Here's how the part is built. I have some questions about the finished solid (model axes, mm). Face numbers are marked on the shaded views. A direction names the side the tool comes from. Give positions to 0.01 mm unless a question says otherwise; leave off trailing zeros. Loops run counter-clockwise (first coordinate to the right, second up) from the corner with the lowest first, then second, coordinate; pieces in that order, holes last. Notation, with made-up numbers: M 4.25,36 L 8.25,36 A20 cw 8.25,67 Z; hole C 3.25,-32 d11. An arc over 180 degrees is marked long. Answer as CSV lines item,"result". Start each with the question number.
Item 1: I want a section at B-B on y = 6.5. List the corners of the cut face in (x, z) for me, plus the area to 3 significant figures.
Item 2: For the marked faces 4, 5 and 6, which set-ups out of +Z, -Z, +X, -X, +Y, -Y let a thin tool reach every point of the face, with its end or its side?
Item 3: I want a section at A-A on z = 2.5. List the corners of the cut face in (x, y) for me, plus the area to 3 significant figures.
Item 4: If I drill on line 1 along Y through (x, z) = (-17, 13.25); line 2 along Y through (x, z) = (2, 10.25); line 3 along X through (y, z) = (-3, 6.5), over which ranges is the centre line in solid material (lowest first)? Write a range as from..to.
Item 5: I want a section at C-C on x = -17. List the corners of the cut face in (y, z) for me.
Item 6: I want a section at D-D on y = -7. List the corners of the cut face in (x, z) for me, plus the area to 3 significant figures.
Item 7: If we mould it in two halves opening along Z, with no side actions, what happens to the marked faces 1, 2 and 3? For each: released by +Z, released by -Z, zero draft, split by the parting line, or undercut.
Item 8: Will these pins go through, and if not, where does the flat tip stop? P1, Ø5, axis at x = 27.5, z = 13, coming from the -Y side; P2, Ø6.5, axis at y = 3.5, z = 8, coming from the +X side; P3, Ø12, axis at x = 29.5, y = -25, coming from the -Z side.
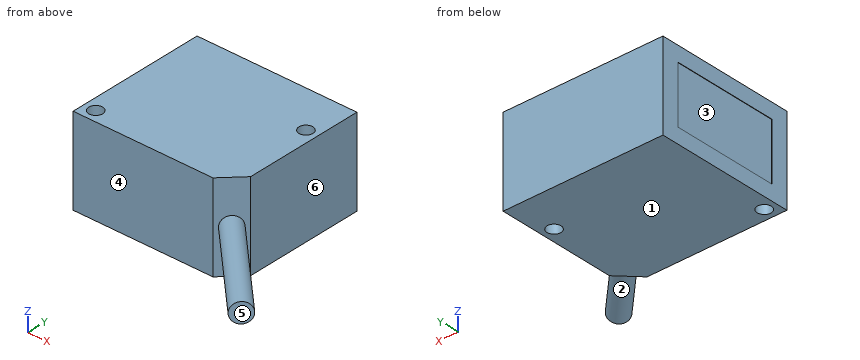
from build123d import *

# Parameters (mm, degrees)
SKETCH_1_W          = 40
SKETCH_1_H          = 35
EXTRUDE_1_DEPTH     = 22
SKETCH_2_R          = 1.75
CUT_EXTRUDE_1_DEPTH = 35.5
CHAMFER_1_SIZE      = 5
SKETCH_3_R          = 2.5
EXTRUDE_2_DEPTH     = 30
SKETCH_4_W          = 14.42354322
SKETCH_4_H          = 26.54144869
CUT_EXTRUDE_2_DEPTH = 0.1


with BuildPart() as part:
    # 草图1 → 凸台-拉伸1 (new body)
    with BuildSketch(Plane.XY):
        Rectangle(SKETCH_1_W, SKETCH_1_H)
    extrude(amount=EXTRUDE_1_DEPTH)

    # 草图2 → 切除-拉伸1 (cut, through all)
    with BuildSketch(Plane.XY.offset(22)):
        with Locations((17, 6.5)):
            Circle(SKETCH_2_R)
        with Locations((-17, -14.5)):
            Circle(SKETCH_2_R)
    extrude(amount=-CUT_EXTRUDE_1_DEPTH, mode=Mode.SUBTRACT)

    # 倒角1
    chamfer_1_edges = [part.edges().sort_by_distance(p)[0] for p in [
        (20, -17.5, 11),
    ]]
    chamfer(chamfer_1_edges, length=CHAMFER_1_SIZE)

    # 草图3 → 凸台-拉伸2 (add)
    with BuildSketch(Plane(origin=(16.25, -16.25, 0), x_dir=(0, 0, -1), z_dir=(0.7071067811865467, -0.7071067811865485, 0))):
        with Locations(Location((-11, 1.767766953, 0), (0, 0, 90))):
            Circle(SKETCH_3_R)
    extrude(amount=EXTRUDE_2_DEPTH)

    # 草图4 → 切除-拉伸2 (cut)
    with BuildSketch(Plane.ZY.offset(20)):
        with Locations((11, 0)):
            Rectangle(SKETCH_4_W, SKETCH_4_H)
    extrude(amount=-CUT_EXTRUDE_2_DEPTH, mode=Mode.SUBTRACT)


solid = part.part
Result:
1,outline,"M -20,0 L 15.25,0 L 15.25,22 L -20,22 L -20,18.21 L -19.9,18.21 L -19.9,3.79 L -20,3.79 Z; M 18.75,0 L 20,0 L 20,22 L 18.75,22 Z"
1,area,"802 mm^2"
2,face 4,"+Z, -Z, -X, -Y"
2,face 5,"+Z, -Z, +X, -Y"
2,face 6,"+Z, -Z, +X, +Y"
3,outline,"M -20,-17.5 L 15,-17.5 L 20,-12.5 L 20,17.5 L -20,17.5 Z; hole C -17,-14.5 d3.5; hole C 17,6.5 d3.5"
3,area,"1,370 mm^2"
4,line 1,"-17.5..-16.25, -12.75..17.5"
4,line 2,"-17.5..17.5"
4,line 3,"-19.9..20"
5,outline,"M -17.5,0 L -16.25,0 L -16.25,22 L -17.5,22 Z; M -12.75,0 L 17.5,0 L 17.5,22 L -12.75,22 Z"
6,outline,"M -20,0 L 20,0 L 20,22 L -20,22 L -20,18.21 L -19.9,18.21 L -19.9,3.79 L -20,3.79 Z"
6,area,"879 mm^2"
7,face 1,"released by -Z"
7,face 2,"split by the parting line"
7,face 3,"undercut"
8,P1,"y = -30.54"
8,P2,"x = 20"
8,P3,"z = 8.5"
